from build123d import *

# Parameters (mm, degrees)
F1_DEPTH = 5
F2_DEPTH = 25
F3_R     = 4.99999


# Not quite as in the source:
# - a fillet or chamfer is up to 0.001 mm smaller than in the source, because OpenCascade refuses the exact size


with BuildPart() as f1:
    # F0 (on Top) → F1 (new body)
    with BuildSketch(Plane.XY):
        with BuildLine():
            add(Edge.make_bspline(
                [(0, 47.6761966849), (31.7996343084, 66.3650460849), (162.4107710873, 1.1493064278), (-0.5654891103, -87.7590913423), (-23.5407682827, -21.5589349291), (-22.8451150266, 0)],
                knots=[0, 0, 0, 0, 0.3365827736, 0.6764560587, 0.845419572, 0.845419572, 0.845419572, 0.845419572], degree=3))
            add(Edge.make_bspline(
                [(-22.8451150266, 0), (-22.2086795266, 19.7237221407), (-14.6044345316, 39.0930766752), (0, 47.6761966849)],
                knots=[0.845419572, 0.845419572, 0.845419572, 0.845419572, 1, 1, 1, 1], degree=3))
        make_face()
        Polygon((-2.4451150266, -24.6), (-2.4451150266, 0), (-2.4451150266, 24.6), (46.7548849734, 24.6), (46.7548849734, -24.6), align=None, mode=Mode.SUBTRACT)
    extrude(amount=F1_DEPTH)

    # F0 (on Top) → F2 (join)
    with BuildSketch(Plane.XY):
        Polygon((-2.4451150266, 24.6), (-2.4451150266, 0), (-2.4451150266, -24.6), (46.7548849734, -24.6), (46.7548849734, 24.6), align=None)
        Polygon((-0.8451150266, -23), (-0.8451150266, 0), (-0.8451150266, 23), (45.1548849734, 23), (45.1548849734, -23), align=None, mode=Mode.SUBTRACT)
    extrude(amount=F2_DEPTH)

    # F3 (radius 5 in the source; OpenCascade refuses exactly that, so slightly less here)
    f3_edges = [f1.edges().sort_by_distance(p)[0] for p in [
        (46.754885, 0, 5),
        (22.154885, -24.6, 5),
        (-2.445115, 0, 5),
        (22.154885, 24.6, 5),
        (84.577965, -27.452992, 5),
    ]]
    fillet(f3_edges, radius=F3_R)


solid = f1.part
Part model, mm, in its own coordinate system. A direction names the side the tool comes from. Give positions to 0.01 mm unless a question says otherwise; leave off trailing zeros. Order: outer loops, then holes, each group sorted by start corner. A loop starts at its lowest first (then second) coordinate and runs counter-clockwise, first axis right, second up. Notation, with made-up numbers: (-1.75, -39) - (55.25, -39) arc R23 cw to (55.25, -3) - close; hole circle Ø2 at (54.25, 19). An arc over 180 degrees is marked (long way). Use a Markdown table: item, result.
1) Probe L1, parallel to X at y = 7.5, z = 23.25; L2, parallel to Y at x = 23, z = 12; L3, parallel to Z at x = 62.5, y = -11.5. List the from-to ranges inside material, lowest first. Write a range as from..to.
Checked values:
| item | result |
|---|---|
| L1 | -2.45..-0.85, 45.15..46.75 |
| L2 | -24.6..-23, 23..24.6 |
| L3 | 0..5 |
2) Flat gauge pins, fed straight in: P1, Ø7.5, axis at x = 28.5, z = 18, coming from the -Y side; P2, Ø12, axis at x = 20, z = 17, coming from the +Y side; P3, Ø10, axis at y = -24.5, z = 10.5, coming from the -X side. Where does each tip first touch, or does it go through?
Checked values:
| item | result |
|---|---|
| P1 | y = -24.6 |
| P2 | y = 24.6 |
| P3 | x = -5.27 |
3) 3-axis set-ups, long thin cutter, end or side, ignore diameter. For faces 4 (the flat face through (-2.445, 0, 17)), 5 (the flat face through (22, -24.6, 17)), 6 (the flat face through (46.755, 0, 17)): which of +Z, -Z, +X, -X, +Y, -Y reach the whole face in a straight line?
Checked values:
| item | result |
|---|---|
| face 4 | +Z, -X, +Y, -Y |
| face 5 | +Z, +X, -X, -Y |
| face 6 | +Z, +X, +Y, -Y |
4) Saw through at A-A on z = 21.25. List the corners of the cut face in (x, y).
Checked values:
| item | result |
|---|---|
| outline | (-2.45, -24.6) - (46.75, -24.6) - (46.75, 24.6) - (-2.45, 24.6) - close; hole (-0.85, -23) - (45.15, -23) - (45.15, 23) - (-0.85, 23) - close |
5) Two-plate mould, pull along X, no slides. Class faces 1 (the cylindrical face through (21.74, -26.1, 6.43)), 2 (the flat face through (22, -23, 12)), 3 (the cylindrical face through (48.258, -0.414, 6.426)): +X half, -X half, draft (parallel to the pull), parting line (faces both ways), or undercut.
Checked values:
| item | result |
|---|---|
| face 1 | draft |
| face 2 | undercut |
| face 3 | +X half |
